Input: part model. Units: mm. Frame: model coordinates. A direction names the side the tool comes from. Coordinates: 2 decimals unless noted, no trailing zeros. Order: outer loops, then holes, each group sorted by start corner. A loop starts at its lowest first (then second) coordinate and runs counter-clockwise, first axis right, second up. Notation, with made-up numbers: (-9, -19) -> (34, -19) arc R10 ccw to (34, -10) -> close; hole circle Ø6 at (31, 15.25). An arc over 180 degrees is marked (long way). Answer as CSV lines item,"result".
from build123d import *

# Parameters (mm, degrees)
SKETCH042_R     = 3.0625
PAD006_DEPTH    = 27.5
SKETCH043_R     = 1.6
POCKET027_DEPTH = 5
POCKET028_DEPTH = 2
SKETCH046_W     = 26
SKETCH046_H     = 8
POCKET029_DEPTH = 14
SKETCH047_W     = 10
SKETCH047_H     = 5.5
PAD007_DEPTH    = 5
SKETCH048_R     = 1.6
POCKET030_DEPTH = 8.5
SKETCH049_W     = 6.5
SKETCH049_H     = 2.5
POCKET031_DEPTH = 6.5
SKETCH050_W     = 6.5
SKETCH050_H     = 2.5
POCKET032_DEPTH = 8.18
FILLET002_R     = 1


with BuildPart() as part:
    # Sketch042 → Pad006 (new body)
    with BuildSketch(Plane.XZ):
        Polygon((33, -7), (33, 2), (75, 2), (75, 7), (-75, 7), (-75, 2), (-33, 2), (-33, -7), (-7, -7), (-7, 2), (7, 2), (7, -7), align=None)
        with Locations((-14, 0)):
            Circle(SKETCH042_R, mode=Mode.SUBTRACT)
        with Locations((14, 0)):
            Circle(SKETCH042_R, mode=Mode.SUBTRACT)
        with Locations((-26, 0)):
            Circle(SKETCH042_R, mode=Mode.SUBTRACT)
        with Locations((26, 0)):
            Circle(SKETCH042_R, mode=Mode.SUBTRACT)
    extrude(amount=PAD006_DEPTH)

    # Sketch043 (on Face4 of Pad006) → Pocket027 (cut)
    with BuildSketch(Plane(origin=(0, 0, 7), x_dir=(-1, 0, 0), z_dir=(0, 0, 1))):
        with Locations((-66.75, 13.75)):
            Circle(SKETCH043_R)
        with Locations((66.75, 13.75)):
            Circle(SKETCH043_R)
    extrude(amount=-POCKET027_DEPTH, mode=Mode.SUBTRACT)

    # Sketch045 (on Face11 of Pocket027) → Pocket028 (cut)
    with BuildSketch(Plane(origin=(0, 0, 2), x_dir=(1, 0, 0), z_dir=(0, 0, -1))):
        Polygon((-63.5, 13.75), (-65.125, 16.5645825623), (-68.375, 16.5645825623), (-70, 13.75), (-68.375, 10.9354174377), (-65.125, 10.9354174377), align=None)
        Polygon((70, 13.75), (68.375, 16.5645825623), (65.125, 16.5645825623), (63.5, 13.75), (65.125, 10.9354174377), (68.375, 10.9354174377), align=None)
    extrude(amount=-POCKET028_DEPTH, mode=Mode.SUBTRACT)

    # Sketch046 (on Face14 of Pocket028) → Pocket029 (cut)
    with BuildSketch(Plane(origin=(0, 0, 7), x_dir=(-1, 0, 0), z_dir=(0, 0, 1))):
        with Locations((-20, 13.5)):
            Rectangle(SKETCH046_W, SKETCH046_H)
        with Locations((20, 13.5)):
            Rectangle(SKETCH046_W, SKETCH046_H)
    extrude(amount=-POCKET029_DEPTH, mode=Mode.SUBTRACT)

    # Sketch047 (on Face7 of Pocket022) → Pad007 (join)
    with BuildSketch(Plane(origin=(0, 0, 7), x_dir=(-1, 0, 0), z_dir=(0, 0, 1))):
        with Locations((-10.16, 23.07)):
            Rectangle(SKETCH047_W, SKETCH047_H)
        with Locations((10.16, 23.07)):
            Rectangle(SKETCH047_W, SKETCH047_H)
        with Locations((-10.16, 2.75)):
            Rectangle(SKETCH047_W, SKETCH047_H)
        with Locations((10.16, 2.75)):
            Rectangle(SKETCH047_W, SKETCH047_H)
    extrude(amount=PAD007_DEPTH)

    # Sketch048 (on Face52 of Pad007) → Pocket030 (cut)
    with BuildSketch(Plane(origin=(0, 0, 12), x_dir=(-1, 0, 0), z_dir=(0, 0, 1))):
        with Locations((-10.16, 23.195)):
            Circle(SKETCH048_R)
        with Locations((-10.16, 2.875)):
            Circle(SKETCH048_R)
        with Locations((10.16, 23.195)):
            Circle(SKETCH048_R)
        with Locations((10.16, 2.875)):
            Circle(SKETCH048_R)
    extrude(amount=-POCKET030_DEPTH, mode=Mode.SUBTRACT)

    # Sketch049 (on Face2 of Pocket030) → Pocket031 (cut)
    with BuildSketch(Plane(origin=(0, 0, 0), x_dir=(1, 0, 0), z_dir=(0, 1, 0))):
        with Locations((-10.16, -5.25)):
            Rectangle(SKETCH049_W, SKETCH049_H)
        with Locations((10.16, -5.25)):
            Rectangle(SKETCH049_W, SKETCH049_H)
    extrude(amount=-POCKET031_DEPTH, mode=Mode.SUBTRACT)

    # Sketch050 (on Face31 of Pocket031) → Pocket032 (cut)
    with BuildSketch(Plane.XZ.offset(27.5)):
        with Locations((-10.16, 5.25)):
            Rectangle(SKETCH050_W, SKETCH050_H)
        with Locations((10.16, 5.25)):
            Rectangle(SKETCH050_W, SKETCH050_H)
    extrude(amount=-POCKET032_DEPTH, mode=Mode.SUBTRACT)

    # Fillet002
    fillet002_edges = [part.edges().sort_by_distance(p)[0] for p in [
        (-13.41, -27.5, 5.25),
        (-6.91, -27.5, 5.25),
        (6.91, -27.5, 5.25),
        (13.41, -27.5, 5.25),
        (13.41, 0, 5.25),
        (6.91, 0, 5.25),
        (-6.91, 0, 5.25),
        (-13.41, 0, 5.25),
    ]]
    fillet(fillet002_edges, radius=FILLET002_R)


solid = part.part
1. Reachability of faces 1 (the face through (-20, -17.5, 0)), 2 (the face through (10, -20.32, 9)), 3 (the face through (10, -5, 4)), 4 (the face through (10, -19.32, 5)) from +Z, -Z, +X, -X, +Y, -Y: full face, straight path, thin tool, end or side. Return the list, or none.
Findings:
face 1,"+Z, -Z"
face 2,"+Z, +X, -X"
face 3,"+Y"
face 4,"-Y"
2. Contact query for flat-ended pins moving along their axis: pin 1 (1.5 mm diameter, centred on y = -23.5, z = 10, fed in from -X); pin 2 (1.5 mm diameter, centred on y = -5, z = 1, fed in from +X); pin 3 (3 mm diameter, centred on x = -10.16, y = -23.195, fed in from +Z); pin 4 (8 mm diameter, centred on x = 4.5, y = -22.5, fed in from -Z). Output: stop coordinate, or through.
Findings:
pin 1,"stops at x = -15.16"
pin 2,"stops at x = 33"
pin 3,"stops at z = 3.5"
pin 4,"stops at z = -7"
3. Mould query, pull axis X, two halves, no side actions, for faces 5 (the face through (20, -5, -7)), 6 (the face through (-8.89, -22.22, 3.75)), 7 (the face through (-15.16, -3, 9)), 8 (the face through (6.91, -23, 5)). Classes: released by +X, released by -X, zero draft, split by the parting line, or undercut.
Findings:
face 5,"zero draft"
face 6,"undercut"
face 7,"released by -X"
face 8,"undercut"
4. Cut plane A-A (x = -21). Return the cut outline in (y, z).
Findings:
outline,"(-27.5, -7) -> (-17.5, -7) -> (-17.5, 7) -> (-27.5, 7) -> close; (-9.5, -7) -> (0, -7) -> (0, 7) -> (-9.5, 7) -> close"
5. Cut plane C-C (x = 66.75). Return the cut outline in (y, z), plus the area to 3 significant figures.
Findings:
outline,"(-27.5, 2) -> (-16.56, 2) -> (-16.56, 4) -> (-15.35, 4) -> (-15.35, 7) -> (-27.5, 7) -> close; (-12.15, 4) -> (-10.94, 4) -> (-10.94, 2) -> (0, 2) -> (0, 7) -> (-12.15, 7) -> close"
area,"117 mm2"
6. Cut plane D-D (z = 0). State how many separate pieces and enclosed holes the cut face has, plus the area to 3 significant figures.
Findings:
separate pieces,"12"
enclosed holes,"0"
area,"536 mm2"
7. Cut plane B-B (z = 8.25). Return the cut outline in (x, y) (3 decimals).
Findings:
outline,"(-15.16, -25.82) -> (-5.16, -25.82) -> (-5.16, -20.32) -> (-15.16, -20.32) -> close; (-15.16, -5.5) -> (-5.16, -5.5) -> (-5.16, 0) -> (-15.16, 0) -> close; (5.16, -25.82) -> (15.16, -25.82) -> (15.16, -20.32) -> (5.16, -20.32) -> close; (5.16, -5.5) -> (15.16, -5.5) -> (15.16, 0) -> (5.16, 0) -> close; hole circle Ø3.2 at (-10.16, -23.195); hole circle Ø3.2 at (-10.16, -2.875); hole circle Ø3.2 at (10.16, -23.195); hole circle Ø3.2 at (10.16, -2.875)"
8. Ray query, line 1 along Y through (x, z) = (-10.16, 10.4) (3 decimals); line 2 along X through (y, z) = (-13.75, 5.5); line 3 along X through (y, z) = (-24.25, 0). Return the intervals inside material, ascending.
Findings:
line 1,"y = -25.82 to -24.795, -21.595 to -20.32, -5.5 to -4.475, -1.275 to 0"
line 2,"x = -75 to -68.35, -65.15 to -33, -7 to 7, 33 to 65.15, 68.35 to 75"
line 3,"x = -33 to -29.06, -22.94 to -17.06, -10.94 to -7, 7 to 10.94, 17.06 to 22.94, 29.06 to 33"
